Read the model definition and answer for the solid it produces. Units are mm, in the model's axes. Face numbers are marked on the shaded views. Round coordinates to 2 decimals unless told otherwise and drop trailing zeros. Loops run counter-clockwise (first coordinate to the right, second up) from the corner with the lowest first, then second, coordinate; pieces in that order, holes last. Notation, with made-up numbers: M 63.25,-38 L 114.25,-38 A25 cw 114.25,-1 Z; hole C 13.5,42.5 d4. An arc over 180 degrees is marked long. Answer as CSV lines item,"result".
```python
from build123d import *

# Parameters (mm, degrees)
F0_R     = 11.05
F1_DEPTH = 3.5
F2_R     = 11.05
F2_R_2   = 9.55
F3_DEPTH = 0.5
F4_R     = 1.5
F5_DEPTH = 2
F6_R     = 0.9
F6_R_2   = 0.9063368872
F7_DEPTH = 2


with BuildPart() as f1:
    # F0 (on Top) → F1 (new body)
    with BuildSketch(Plane.XY):
        with BuildLine():
            ThreePointArc((-2.4893394798, 39.5443588099), (-10.4243237179, 34.8815428811), (-13.55, 26.2249861161))
            Line((-13.55, 26.2249861161), (-13.55, 7.0192147502))
            Line((-13.55, 7.0192147502), (-30.1826859022, -2.5836709328))
            ThreePointArc((-30.1826859022, -2.5836709328), (-36.1166458289, -9.6188643795), (-36.1872707573, -18.8221702728))
            ThreePointArc((-36.1872707573, -18.8221702728), (-35.1423301235, -21.093315154), (-33.6979312775, -23.133832729))
            ThreePointArc((-33.6979312775, -23.133832729), (-25.692322111, -27.6743226935), (-16.6326859022, -26.0529593753))
            Line((-16.6326859022, -26.0529593753), (0, -16.4500736924))
            Line((0, -16.4500736924), (16.6326859022, -26.0529593753))
            ThreePointArc((16.6326859022, -26.0529593753), (25.692322111, -27.6743226935), (33.6979312775, -23.133832729))
            ThreePointArc((33.6979312775, -23.133832729), (35.1423301235, -21.093315154), (36.1872707573, -18.8221702728))
            ThreePointArc((36.1872707573, -18.8221702728), (36.1166458289, -9.6188643795), (30.1826859022, -2.5836709328))
            Line((30.1826859022, -2.5836709328), (13.55, 7.0192147502))
            Line((13.55, 7.0192147502), (13.55, 26.2249861161))
            ThreePointArc((13.55, 26.2249861161), (10.4243237179, 34.8815428811), (2.4893394798, 39.5443588099))
            ThreePointArc((2.4893394798, 39.5443588099), (0, 39.7749861161), (-2.4893394798, 39.5443588099))
        make_face()
        with Locations((-23.4076859022, -14.318315154)):
            Circle(F0_R, mode=Mode.SUBTRACT)
        with Locations((0, -0.7750138839)):
            Circle(F0_R, mode=Mode.SUBTRACT)
        with Locations((23.4076859022, -14.318315154)):
            Circle(F0_R, mode=Mode.SUBTRACT)
        with Locations((0, 26.2249861161)):
            Circle(F0_R, mode=Mode.SUBTRACT)
        with BuildLine():
            ThreePointArc((2.4893394798, 39.5443588099), (0, 42.2749861161), (-2.4893394798, 39.5443588099))
            ThreePointArc((-2.4893394798, 39.5443588099), (0, 39.7749861161), (2.4893394798, 39.5443588099))
        make_face()
        with BuildLine():
            ThreePointArc((-33.6979312775, -23.133832729), (-35.1423301235, -21.093315154), (-36.1872707573, -18.8221702728))
            ThreePointArc((-36.1872707573, -18.8221702728), (-37.3073936329, -22.343315154), (-33.6979312775, -23.133832729))
        make_face()
        with BuildLine():
            ThreePointArc((33.6979312775, -23.133832729), (37.3073936329, -22.343315154), (36.1872707573, -18.8221702728))
            ThreePointArc((36.1872707573, -18.8221702728), (35.1423301235, -21.093315154), (33.6979312775, -23.133832729))
        make_face()
    extrude(amount=F1_DEPTH)

    # F2 (on face) → F3 (join)
    with BuildSketch(Plane.XY.offset(3.5)):
        with BuildLine():
            Line((13.55, 7.0192147502), (13.55, 26.2249861161))
            ThreePointArc((13.55, 26.2249861161), (10.4243237179, 34.8815428811), (2.4893394798, 39.5443588099))
            ThreePointArc((2.4893394798, 39.5443588099), (0, 42.2749861161), (-2.4893394798, 39.5443588099))
            ThreePointArc((-2.4893394798, 39.5443588099), (-10.4243237179, 34.8815428811), (-13.55, 26.2249861161))
            Line((-13.55, 26.2249861161), (-13.55, 7.0192147502))
            Line((-13.55, 7.0192147502), (-30.1826859022, -2.5836709328))
            ThreePointArc((-30.1826859022, -2.5836709328), (-36.1166458289, -9.6188643795), (-36.1872707573, -18.8221702728))
            ThreePointArc((-36.1872707573, -18.8221702728), (-37.3073936329, -22.343315154), (-33.6979312775, -23.133832729))
            ThreePointArc((-33.6979312775, -23.133832729), (-25.692322111, -27.6743226935), (-16.6326859022, -26.0529593753))
            Line((-16.6326859022, -26.0529593753), (0, -16.4500736924))
            Line((0, -16.4500736924), (16.6326859022, -26.0529593753))
            ThreePointArc((16.6326859022, -26.0529593753), (25.692322111, -27.6743226935), (33.6979312775, -23.133832729))
            ThreePointArc((33.6979312775, -23.133832729), (37.3073936329, -22.343315154), (36.1872707573, -18.8221702728))
            ThreePointArc((36.1872707573, -18.8221702728), (36.1166458289, -9.6188643795), (30.1826859022, -2.5836709328))
            Line((30.1826859022, -2.5836709328), (13.55, 7.0192147502))
        make_face()
        with Locations((-23.4076859022, -14.318315154)):
            Circle(F2_R, mode=Mode.SUBTRACT)
        with Locations((0, -0.7750138839)):
            Circle(F2_R, mode=Mode.SUBTRACT)
        with Locations((23.4076859022, -14.318315154)):
            Circle(F2_R, mode=Mode.SUBTRACT)
        with Locations((0, 26.2249861161)):
            Circle(F2_R, mode=Mode.SUBTRACT)
        with Locations((0, 26.2249861161)):
            Circle(F2_R)
        with Locations((0, 26.2249861161)):
            Circle(F2_R_2, mode=Mode.SUBTRACT)
        with Locations((0, -0.7750138839)):
            Circle(F2_R)
        with Locations((0, -0.7750138839)):
            Circle(F2_R_2, mode=Mode.SUBTRACT)
        with Locations((-23.4076859022, -14.318315154)):
            Circle(F2_R)
        with Locations((-23.4076859022, -14.318315154)):
            Circle(F2_R_2, mode=Mode.SUBTRACT)
        with Locations((23.4076859022, -14.318315154)):
            Circle(F2_R)
        with Locations((23.4076859022, -14.318315154)):
            Circle(F2_R_2, mode=Mode.SUBTRACT)
    extrude(amount=F3_DEPTH)

    # F4 (on face) → F5 (cut)
    with BuildSketch(Plane.XY.offset(4)):
        with Locations((0, 39.7749861161)):
            Circle(F4_R)
        with Locations((-35.1423301235, -21.093315154)):
            Circle(F4_R)
        with Locations((35.1423301235, -21.093315154)):
            Circle(F4_R)
        with Locations((0, 12.8714358434)):
            Circle(F4_R)
        with Locations((-11.1469904236, -6.4357179217)):
            Circle(F4_R)
        with Locations((11.1469904236, -6.4357179217)):
            Circle(F4_R)
    extrude(amount=-F5_DEPTH, mode=Mode.SUBTRACT)

    # F6 (on face) → F7 (cut, through all)
    with BuildSketch(Plane.XY.offset(2)):
        with Locations((0, 39.7749861161)):
            Circle(F6_R)
        with Locations((0, 12.8714358434)):
            Circle(F6_R)
        with Locations((-11.1469904236, -6.4357179217)):
            Circle(F6_R_2)
        with Locations((-35.1423301235, -21.093315154)):
            Circle(F6_R_2)
        with Locations((11.1469904236, -6.4357179217)):
            Circle(F6_R_2)
        with Locations((35.1423301235, -21.093315154)):
            Circle(F6_R_2)
    extrude(amount=-F7_DEPTH, mode=Mode.SUBTRACT)


solid = f1.part
```
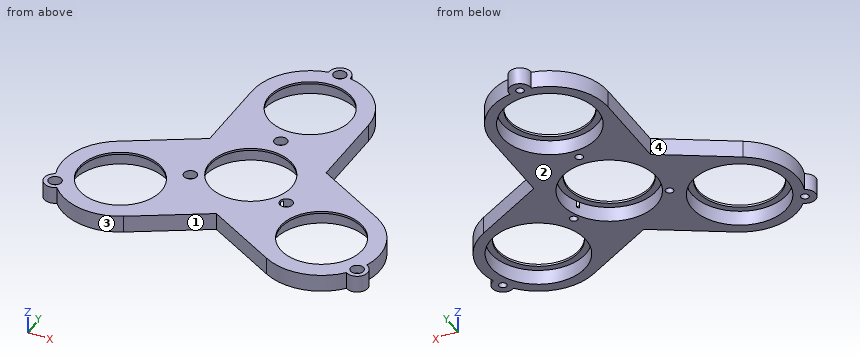
1) Find section A-A, the plane x = 26.5. Give the vertices of the cut face in (y, z).
Evaluation:
outline,"M -27.51,0 L -24.93,0 L -24.93,3.5 L -23.35,3.5 L -23.35,4 L -27.51,4 Z; M -5.28,3.5 L -3.71,3.5 L -3.71,0 L -0.46,0 L -0.46,4 L -5.28,4 Z"
2) Determine the mould class of the marked faces 1, 2, 3 and 4 for opening direction X: released by +X, released by -X, zero draft, split by the parting line, or undercut.
Evaluation:
face 1,"undercut"
face 2,"zero draft"
face 3,"undercut"
face 4,"released by -X"
3) Each of these flat-tipped pins is pushed along its axis until it touches: P1, Ø0.9, axis at x = -35, y = -22, coming from the +Z side; P2, Ø2, axis at y = 17.5, z = 3, coming from the -X side; P3, Ø11, axis at x = -26.5, y = -10.5, coming from the -Z side. Where does it stop, or does it pass through?
Evaluation:
P1,"stops at z = 2"
P2,"stops at x = -13.55"
P3,"stops at z = 3.5"
4) Find section B-B, the plane y = 23.5. Give the vertices of the cut face in (x, z).
Evaluation:
outline,"M -13.55,0 L -10.71,0 L -10.71,3.5 L -9.15,3.5 L -9.15,4 L -13.55,4 Z; M 9.15,3.5 L 10.71,3.5 L 10.71,0 L 13.55,0 L 13.55,4 L 9.15,4 Z"
5) Straight lines are drawn through the part: line 1 (Y direction, x = 0, z = 3.6); line 2 (X direction, y = -8, z = 2); line 3 (X direction, y = -16.5, z = 3.3). For each, find the intervals that lie inside material, in ascending order.
Evaluation:
line 1,"y = -16.45 to -10.33, 8.77 to 11.37, 14.37 to 16.67, 35.77 to 38.27, 41.27 to 42.27"
line 2,"x = -35.39 to -32.47, -14.34 to -8.36, 8.36 to 14.34, 32.47 to 35.39"
line 3,"x = -36.78 to -34.24, -12.58 to -0.09, 0.09 to 12.58, 34.24 to 36.78"
6) Find section C-C, the plane x = 3.5. Give the vertices of the cut face in (y, z).
Evaluation:
outline,"M -18.47,0 L -11.26,0 L -11.26,3.5 L -9.66,3.5 L -9.66,4 L -18.47,4 Z; M 8.11,3.5 L 9.71,3.5 L 9.71,0 L 15.74,0 L 15.74,3.5 L 17.34,3.5 L 17.34,4 L 8.11,4 Z; M 35.11,3.5 L 36.71,3.5 L 36.71,0 L 39.32,0 L 39.32,4 L 35.11,4 Z"
